Build history of the part. All positions in model axes, mm. A direction names the side the tool comes from. Coordinates: 2 decimals unless noted, no trailing zeros. Loops run counter-clockwise (first coordinate to the right, second up) from the corner with the lowest first, then second, coordinate; pieces in that order, holes last. Notation, with made-up numbers: M 73,-35.5 L 130,-35.5 A27 cw 130,-14.5 Z; hole C -23.5,18 d3. An arc over 180 degrees is marked long. Write each question's results on one line, items separated by ' | '. Start each with the question number.
from build123d import *

# Parameters (mm, degrees)
F0_W      = 50
F0_H      = 12.5
F1_DEPTH  = 8
F2_DEPTH  = 75
F4_DEPTH  = 8
F7_DEPTH  = 3
F8_DEPTH  = 1
F11_DEPTH = 3
F14_DEPTH = 3
F15_DEPTH = 8
F16_DEPTH = 8
F17_DEPTH = 8


with BuildPart() as f1:
    # F0 (on Top) → F1 (new body)
    with BuildSketch(Plane.XY):
        Polygon((-42.0179491924, 72.7772228311), (-60.5095952989, 40.7487522591), (-57.9695070384, 39.3207329262), (-55.5194165334, 43.6791064608), (-50.2642610162, 40.7248836223), (-52.7144317239, 36.366367418), (-57.615009792, 27.6494680496), (-60.0654171506, 23.2910848888), (-65.3204122546, 26.2455930623), (-62.870004896, 30.6039762231), (-65.5097997054, 32.0881441788), (-84.0358983849, 0), (-42.0179491924, -72.7772228311), (42.0179491924, -72.7772228311), (84.0358983849, 0), (65.5097997054, 32.0881441788), (62.870004896, 30.6039762231), (65.3204122546, 26.2455930623), (60.0654171506, 23.2910848888), (57.615009792, 27.6494680496), (55.164720758, 32.0079177338), (52.7144317239, 36.366367418), (50.2642610162, 40.7248836223), (55.5194165334, 43.6791064608), (57.9695070384, 39.3207329262), (60.5095952989, 40.7487522591), (42.0179491924, 72.7772228311), align=None)
        with Locations((0, 54.5829171234)):
            Rectangle(F0_W, F0_H, mode=Mode.SUBTRACT)
    extrude(amount=F1_DEPTH)

    # F0 (on Top) → F2 (join)
    with BuildSketch(Plane.XY):
        Polygon((68.1246734519, -33.5590499945), (87.5, 0), (84.0358983849, 0), (42.0179491924, -72.7772228311), (-42.0179491924, -72.7772228311), (-84.0358983849, 0), (-87.5, 0), (-68.1246734519, -33.5590499945), (-63.1745123486, -42.1329805311), (-43.75, -75.7772228311), (43.75, -75.7772228311), (63.1745123486, -42.1329805311), align=None)
    extrude(amount=F2_DEPTH)

    # F0 (on Top) → F4 (join)
    with BuildSketch(Plane.XY):
        Polygon((43.75, 75.7772228311), (-43.75, 75.7772228311), (-63.1248363216, 42.2190219338), (-60.5095952989, 40.7487522591), (-42.0179491924, 72.7772228311), (42.0179491924, 72.7772228311), (60.5095952989, 40.7487522591), (63.1248363216, 42.2190219338), align=None)
    extrude(amount=F4_DEPTH)

    # F6 (on face) → F7 (join)
    with BuildSketch(Plane(origin=(0, -50.1312366318, 89.3836679776), x_dir=(1, 0, 0), z_dir=(0, 0.4891706574, -0.872188092))):
        Polygon((43.75, 29.4041920927), (0, 29.4041920927), (-43.75, 29.4041920927), (-42.01795, -57.4775522498), (42.01795, -57.4775522498), align=None)
    extrude(amount=F7_DEPTH)

    # F3 (on Front) → F8 (join)
    with BuildSketch(Plane.XZ):
        Polygon((-42.01795, 114.5), (0, 114.5), (42.01795, 114.5), (84.0359, 75), (87.5, 75), (42.01795, 117.5), (0, 117.5), (-42.01795, 117.5), (-87.5, 75), (-84.0359, 75), align=None)
    extrude(amount=F8_DEPTH)

    # F10 (on face) → F11 (join)
    with BuildSketch(Plane(origin=(-67.6846727043, -39.0777640058, 72.4338274863), x_dir=(0.7723629594, -0.3015876344, 0.5590173143), z_dir=(-0.6351814378, -0.3667221741, 0.6797495039))):
        Polygon((33.2314262259, 55.789645187), (-25.6554603702, 35.6104118215), (30.9888924807, -31.0804218073), align=None)
    extrude(amount=-F11_DEPTH)

    # F13 (on face) → F14 (join)
    with BuildSketch(Plane(origin=(67.6756688636, -39.5950852503, 72.4241918832), x_dir=(0.7733047167, 0.3041472681, -0.556322078), z_dir=(-0.6340345536, 0.3709553614, -0.6785221475))):
        Polygon((-30.939509805, 30.5117392321), (-32.8751652468, -56.3649154418), (25.9400068576, -35.9776056011), align=None)
    extrude(amount=F14_DEPTH)

    # F0 (on Top) → F15 (join)
    with BuildSketch(Plane.XY):
        with Locations((0, 54.5829171234)):
            Rectangle(F0_W, F0_H)
    extrude(amount=F15_DEPTH)

    # F0 (on Top) → F16 (join)
    with BuildSketch(Plane.XY):
        Polygon((-78.4478092981, -39.6772904524), (-73.3299584755, -36.6440801541), (-75.878553621, -32.3439069124), (-80.9460908184, -35.4620099819), align=None)
        Polygon((-63.1745123486, -42.1329805311), (-68.1246734519, -33.5590499945), (-73.3299584755, -36.6440801541), (-78.4478092981, -39.6772904524), (-73.3985163623, -48.1928433322), (-68.2616414678, -45.1481695385), align=None)
        Polygon((-65.7363801019, -49.4055813149), (-68.2616414678, -45.1481695385), (-73.3985163623, -48.1928433322), (-70.880193178, -52.396181094), align=None)
        Polygon((75.878553621, -32.3439069124), (73.3299584755, -36.6440801541), (78.4478092981, -39.6772904524), (80.9460908184, -35.4620099819), align=None)
        Polygon((73.3299584755, -36.6440801541), (68.1246734519, -33.5590499945), (63.1745123486, -42.1329805311), (68.2616414678, -45.1481695385), (73.3985163623, -48.1928433322), (78.4478092981, -39.6772904524), align=None)
        Polygon((73.3985163623, -48.1928433322), (68.2616414678, -45.1481695385), (65.7363801019, -49.4055813149), (70.880193178, -52.396181094), align=None)
    extrude(amount=F16_DEPTH)

    # F0 (on Top) → F17 (join)
    with BuildSketch(Plane.XY):
        Polygon((-65.625, 32.1529130712), (-68.125, 33.5584843966), (-87.5, 0), (-84.0358983849, 0), (-65.5097997054, 32.0881441788), align=None)
        Polygon((87.5, 0), (68.125, 33.5584843966), (65.5097997054, 32.0881441788), (84.0358983849, 0), align=None)
    extrude(amount=F17_DEPTH)


solid = f1.part
1. Band-saw the part on B-B, the plane y = -62. List the corners of the cut face in (x, z) (3 decimals).
2. Which spindle directions (+Z, -Z, +X, -X, +Y, -Y) get a long thin tool onto all of the face, cutting with end or side? Do faces 4 (the flat face through (-72, -42, 8)), 5 (the flat face through (-78.377, -33.881, 3.944)), 6 (the flat face through (-74.6, -34.5, 3.9)). Say none if no direction does.
3. Mould opens along Z. For faces 1 (the flat face through (1, -72.777, 40)), 2 (the flat face through (-0.612, -38.912, 95.676)), 3 (the flat face through (1, 75.777, 4)) say: +Z half, -Z half, draft (parallel to the pull), parting line (faces both ways), or undercut.
4. Band-saw the part on A-A, the plane z = 14.5. List the corners of the cut face in (x, y).
5. Band-saw the part on C-C, the plane x = -36. List the corners of the cut face in (y, z).
6. Pin check, flat tips, straight feed: pin 1 (19.5 mm diameter, centred on x = -73, y = -39.5, fed in from +Z); pin 2 (2 mm diameter, centred on x = 18, y = -16.5, fed in from -Z); pin 3 (9 mm diameter, centred on x = 68, y = -44.5, fed in from +Z); pin 4 (3 mm diameter, centred on x = 85, z = 28.5, fed in from +Y). Stop position of each tip, or through.
7. Band-saw the part on D-D, the plane y = -10. List the corners of the cut face in (x, z), plus the area to 3 significant figures.
8. Wall check: line 1 along Z through (x, y) = (-42, -18); line 2 along Z through (x, y) = (53.5, 33.5); line 3 along Z through (x, y) = (-36, -24). Give the ranges that are in metal, low to high.
Checked values:
1) outline: M -51.704,0 L 51.704,0 L 51.704,75 L 51.762,75.046 L 43.477,82.787 L 43.435,82.727 L -43.435,82.727 L -51.704,75 Z; hole M -48.24,8 L 48.24,8 L 48.24,73.915 L 42.491,79.287 L -42.393,79.287 L -48.24,73.824 Z
2) face 4: +Z, -X, -Y | face 5: +Z, -Z, -X | face 6: +Z, -Z
3) face 1: undercut | face 2: +Z half | face 3: draft
4) outline: M -87.5,0 L -43.75,-75.78 L 43.75,-75.78 L 87.5,0 L 84.04,0 L 42.02,-72.78 L -42.02,-72.78 L -84.04,0 Z
5) outline: M -75.78,0 L 75.78,0 L 75.78,8 L -72.78,8 L -72.78,73.24 L 1.47,114.88 L 0,117.5 L -1,117.5 L -1,116.94 L -75.78,75 Z
6) pin 1: z = 77.76 | pin 2: z = 0 | pin 3: z = 8 | pin 4: y = 0
7) outline: M -81.73,0 L 81.73,0 L 81.73,75 L 82,75.22 L 42.45,112.18 L 42.25,111.89 L -42.25,111.89 L -81.73,75 Z; hole M -78.26,8 L 78.26,8 L 78.26,74.29 L 41.7,108.45 L -41.2,108.45 L -78.26,73.82 Z | area: 2,390 mm²
8) line 1: 0 to 8, 103.39 to 107.4 | line 2: 0 to 8 | line 3: 0 to 8, 100.6 to 104.04
